Source: CAD feature listing. Evaluate the final solid. Frame: model axes, mm. Face numbers are marked on the shaded views. A direction names the side the tool comes from. Give positions to 0.01 mm unless a question says otherwise; leave off trailing zeros. Order: outer loops, then holes, each group sorted by start corner. A loop starts at its lowest first (then second) coordinate and runs counter-clockwise, first axis right, second up. Notation, with made-up numbers: M 62.5,54 L 117.5,54 A9 ccw 117.5,66 Z; hole C -1,49.5 d9. An arc over 180 degrees is marked long. Use CSV: the item, a comma, the result in double quotes. Start each with the question number.
Item 1: Section query C-C on z = 26.5. Return loops of the section in (x, y).
Item 2: Section query B-B on x = 35.5. Return loops of the section in (y, z), and give its area (3 significant figures).
Item 3: Section query D-D on z = 52. Return loops of the section in (x, y), and give its area (3 significant figures).
Item 4: Access query for the marked faces 1 and 2. Directions: +Z, -Z, +X, -X, +Y, -Y. A direction counts if a zero-diameter tool reaches every point of the face in a straight line with its end or side. Return the directions, or none.
Item 5: Section query A-A on y = 23.5. Return loops of the section in (x, z).
Item 6: First-contact query: pin 1 (3.5 mm diameter, centred on x = 50.5, z = 62, fed in from -Y); pin 2 (10 mm diameter, centred on y = 16.5, z = 55, fed in from +X); pin 3 (10 mm diameter, centred on y = 15.5, z = 30, fed in from +X). Flat tips, straight axial feed; report the tip coordinate or a pass-through.
Item 7: Ray query, probe 1 along X at (y, z) = (10.5, 11); probe 2 along Y at (x, z) = (8.5, 37); probe 3 along Z at (x, y) = (50, -1.5). Return the intervals inside material, ascending. Write a range as from..to.
from build123d import *

# Parameters (mm, degrees)
SKETCH_1_R               = 2.5
SKETCH_1_R_2             = 1.3
EXTRUDE_1_DEPTH          = 25
EXTRUDE_2_DEPTH          = 25
EXTRUDE_3_DEPTH          = 8
EXTRUDE_3_DEPTH_BACK     = 33
EXTRUDE_4_DEPTH          = 5
SKETCH_4_R               = 1.3
CUT_EXTRUDE_1_DEPTH      = 92.24177093
CUT_EXTRUDE_1_DEPTH_BACK = 92.24177093
SKETCH_7_W               = 3
SKETCH_7_H               = 30
SKETCH_7_W_2             = 2.545959886
CUT_EXTRUDE_2_DEPTH      = 88.173473517
CUT_EXTRUDE_2_DEPTH_BACK = 9
CHAMFER_1_SIZE           = 1


with BuildPart() as part:
    # 草图1 → 凸台-拉伸1 (new body)
    with BuildSketch(Plane(origin=(0, 0, 0), x_dir=(1, 0, 0), z_dir=(0, 1, 0))):
        with Locations(Location((0, 0, 0), (0, 0, 270))):
            Circle(SKETCH_1_R)
        with Locations(Location((0, 0, 0), (0, 0, 270))):
            Circle(SKETCH_1_R_2, mode=Mode.SUBTRACT)
    extrude(amount=EXTRUDE_1_DEPTH)

    # 草图2 → 凸台-拉伸2 (add)
    with BuildSketch(Plane(origin=(0, 25, 0), x_dir=(1, 0, 0), z_dir=(0, 1, 0))):
        with BuildLine():
            ThreePointArc((2.5, 0), (0, -2.5), (-2.5, 0))
            Line((-2.5, 0), (-2.5, -30))
            ThreePointArc((-2.5, -30), (-1.63067791, -32.006781425), (0, -33.464101615))
            Line((0, -33.464101615), (51.335686519, -64.362639487))
            Line((51.335686519, -64.362639487), (53.961524227, -60))
            Line((53.961524227, -60), (2.5, -29.025721421))
            Line((2.5, -29.025721421), (2.5, 0))
        make_face()
    extrude(amount=-EXTRUDE_2_DEPTH)

    # 草图3 → 凸台-拉伸3 (add, two sides)
    with BuildSketch(Plane(origin=(0, 25, 0), x_dir=(1, 0, 0), z_dir=(0, 1, 0))) as extrude_3_sk:
        with BuildLine():
            Line((53.961524227, -60), (51.335686519, -64.362639487))
            ThreePointArc((51.335686519, -64.362639487), (54.829925117, -63.494238598), (53.961524227, -60))
        make_face()
    extrude(amount=EXTRUDE_3_DEPTH)
    extrude(extrude_3_sk.sketch, amount=-EXTRUDE_3_DEPTH_BACK)

    # 草图5 → 凸台-拉伸4 (add)
    with BuildSketch(Plane(origin=(-14.785406604, 0, 24.564883997), x_dir=(0.8567769491001666, 0, 0.5156871721214431), z_dir=(-0.5156871721214431, 0, 0.8567769491001666))):
        Polygon((77.174220423, 25), (77.174220423, 33), (47.215614176, 25), align=None)
    extrude_4 = extrude(amount=-EXTRUDE_4_DEPTH)

    # 镜向1: 凸台-拉伸4 across plane
    add(extrude_4.mirror(Plane(origin=(0, 12.5, 0), x_dir=(0, 0, 1), z_dir=(0, -1, 0))))

    # 草图4 → 切除-拉伸1 (cut, two sides)
    with BuildSketch(Plane(origin=(0, 25, 0), x_dir=(1, 0, 0), z_dir=(0, 1, 0))) as cut_extrude_1_sk:
        with Locations(Location((52.648605373, -62.181319744, 0), (0, 0, 238.956602405))):
            Circle(SKETCH_4_R)
    extrude(amount=CUT_EXTRUDE_1_DEPTH, mode=Mode.SUBTRACT)
    extrude(cut_extrude_1_sk.sketch, amount=-CUT_EXTRUDE_1_DEPTH_BACK, mode=Mode.SUBTRACT)

    # 草图7 → 切除-拉伸2 (cut, two sides)
    with BuildSketch(Plane(origin=(-14.785406604, 0, 24.564883997), x_dir=(0.8567769491001666, 0, 0.5156871721214431), z_dir=(-0.5156871721214431, 0, 0.8567769491001666))) as cut_extrude_2_sk:
        with Locations((75.674220423, 12.5)):
            Rectangle(SKETCH_7_W, SKETCH_7_H)
        with Locations((78.447200366, 12.5)):
            Rectangle(SKETCH_7_W_2, SKETCH_7_H)
    extrude(amount=CUT_EXTRUDE_2_DEPTH, mode=Mode.SUBTRACT)
    extrude(cut_extrude_2_sk.sketch, amount=-CUT_EXTRUDE_2_DEPTH_BACK, mode=Mode.SUBTRACT)

    # 倒角1
    chamfer_1_edges = [part.edges().sort_by_distance(p)[0] for p in [
        (48.765355672, 12.5, 62.815577971),
        (51.39119338, 12.5, 58.452938484),
    ]]
    chamfer(chamfer_1_edges, length=CHAMFER_1_SIZE)


solid = part.part
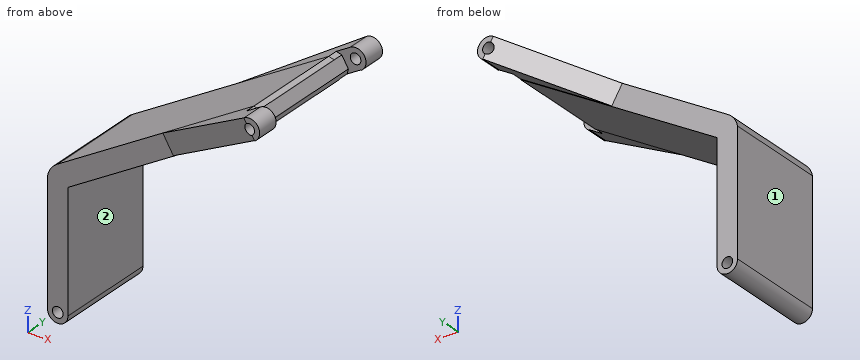
Verdict:
1,outline,"M -2.5,0 L 2.5,0 L 2.5,25 L -2.5,25 Z"
2,outline,"M -3.06,54.83 L -2.26,49 L 0,49 L 0,48.89 L 25,48.89 L 25,49 L 27.26,49 L 28.06,54.83 Z"
2,area,"180 mm2"
3,outline,"M 30.8,-1.6 L 40.49,-3.82 L 40.49,0 L 40.67,0 L 40.67,25 L 40.49,25 L 40.49,28.82 L 30.8,26.6 Z"
3,area,"299 mm2"
4,face 1,"+Z, -Z, -X, +Y, -Y"
4,face 2,"-Z, +X, +Y, -Y"
5,outline,"M -2.5,0 A2.5 ccw 2.5,0 L 2.5,29.03 L 50.53,57.94 L 50.88,59.31 L 49.28,61.96 L 47.91,62.3 L 0,33.46 A5.09 ccw -2.5,30 Z; hole C 0,0 d2.6"
6,pin 1,"y = -7.94"
6,pin 2,"x = 50.88"
6,pin 3,"x = 12.43"
7,probe 1,"-2.5..2.5"
7,probe 2,"0..25"
7,probe 3,"57.72..60.76"
